Autodesk Inventor part; units mm, degrees
ref_plane "YZ Plane" through (0, 0, 0) normal (1, 0, 0) x (0, 1, 0)
ref_plane "XZ Plane" through (0, 0, 0) normal (0, 1, 0) x (-1, 0, 0)
ref_plane "XY Plane" through (0, 0, 0) normal (0, 0, 1) x (1, 0, 0)
sketch "Sketch1" plane through (0, 0, 0) normal (0, 1, 0) x (-1, 0, 0)
  circle A0 centre (0, 0) radius 15
  circle A1 centre (12.3744, 0) radius 1.5
  circle A2 centre (0, 12.3744) radius 1.5
  circle A3 centre (-12.3744, 0) radius 1.5
  circle A4 centre (0, -12.3744) radius 1.5
  dimension "d0" = 30
  dimension "d1" = 3
  dimension "d5" = 360
  dimension "d17" = 14.5
extrude "Extrusion1" add sketch "Sketch1" along normal blind 8
sketch "Sketch2" plane through (0, 8, 0) normal (0, 1, 0) x (1, 0, 0)
  circle A0 centre (0, 0) radius 30
  dimension "d9" = 60
extrude "Extrusion2" add sketch "Sketch2" along normal blind 20
fillet "Fillet1" radius 10 1 edges at (-30, 28, 0)
sketch "Sketch3" plane through (0, 28, 0) normal (0, 1, 0) x (1, 0, 0)
  circle A0 centre (0, 0) radius 1.75
  dimension "d13" = 3.5
extrude "Extrusion3" add sketch "Sketch3" along normal blind 5
fillet "Fillet2" radius 1 2 edges at (-1.75, 28, 0) (-1.75, 33, 0)
equation "\"d0\" = BottomDiameter"
equation "\"d1\" = MountingHoleDiameter"
equation "\"d7\" = BottomHeight"
equation "\"d9\" = TopDiameter"
equation "\"d10\" = TopHeight"
equation "\"d14\" = NubHeight"
equation "\"BottomDiameter\" = 30"
equation "\"MountingHoleDiameter\" = 3"
equation "\"TopDiameter\" = 60"
equation "\"BottomHeight\" = 8"
equation "\"TopHeight\" = 20"
equation "\"NubHeight\" = 5"
properties part number "Motor"
Here's how the part is built. I have some questions about the finished solid (model axes, mm). A direction names the side the tool comes from. Give positions to 0.01 mm unless a question says otherwise; leave off trailing zeros. Loops run counter-clockwise (first coordinate to the right, second up) from the corner with the lowest first, then second, coordinate; pieces in that order, holes last. Notation, with made-up numbers: (63, 82) -> (108, 82) arc R22 cw to (108, 117) -> close; hole circle Ø6 at (60, 77.5). An arc over 180 degrees is marked (long way). One line per item, written item: value.
Q1. We'd pull the mould along Z, two halves only. Please class faces 4 (the face through (13.873, 3.944, -0.066)), 5 (the face through (14.985, 3.944, -0.66)), 6 (the face through (0, 0, 0)): pulls with the +Z half, pulls with the -Z half, needs draft (parallel to the pull), parting line crosses it, or undercut.
Answers follow:
face 4: undercut
face 5: parting line crosses it
face 6: needs draft
Q2. Suppose I cut it at A-A on y = 11. Please give me the cut outline in (x, z).
Answers follow:
outline: circle Ø60 at (0, 0)
Q3. On a 3-axis mill with a long thin cutter (end or side, diameter ignored), from which of +Z, -Z, +X, -X, +Y, -Y can I reach the whole of each face in a straight line? I mean faces 1 (the face through (1.617, 30.479, -0.67)), 2 (the face through (-29.97, 12.93, 1.32)), 3 (the face through (0, 8, 12)). Say none if no direction works.
Answers follow:
face 1: +Y
face 2: +Y, -Y
face 3: -Y
Q4. If I drill on line 1 along Z through (x, y) = (0, 3.5); line 2 along Y through (x, z) = (-5, -6.5); line 3 along Y through (x, z) = (9.5, -12.5), over which ranges is the centre line in solid material (lowest first)?
Answers follow:
line 1: -15 to -13.87, -10.87 to 10.87, 13.87 to 15
line 2: 0 to 28
line 3: 8 to 28
Q5. I'm going to push flat-ended pins straight in: pin 1 Ø5 at (y, z) = (4.5, 8.5) entering from -X; pin 2 Ø4 at (x, z) = (19.5, -6) entering from +Y; pin 3 Ø2.5 at (x, z) = (0, 12.37) entering from -Y; pin 4 Ø2.5 at (x, z) = (-12.5, 0.5) entering from -Y. Where does each tip first touch, or does it pass through?
Answers follow:
pin 1: x = -13.75
pin 2: y = 28
pin 3: y = 8
pin 4: y = 0
Q6. Suppose I cut it at B-B on y = 24. Please give me the cut outline in (x, z).
Answers follow:
outline: circle Ø56 at (0, 0)
